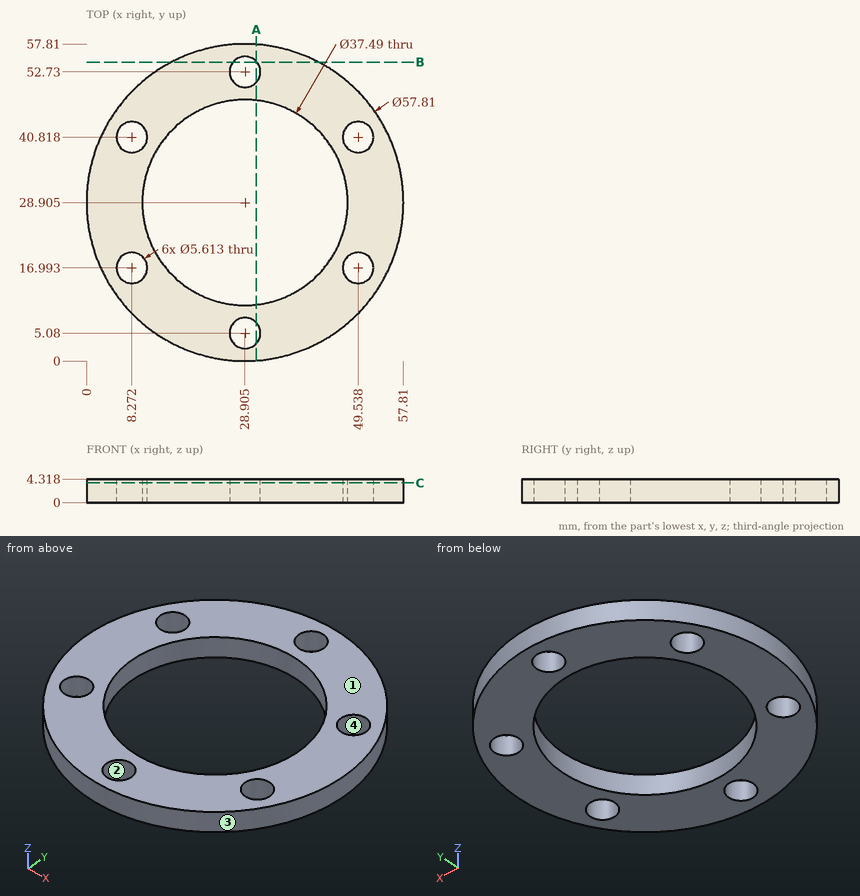
Check sheet for the drawn part. Datum: minimum x, y, z corner. Units: mm. Give positions to 0.01 mm unless a question says otherwise; leave off trailing zeros. Loops run counter-clockwise (first coordinate to the right, second up) from the corner with the lowest first, then second, coordinate; pieces in that order, holes last.
1) Depth check by flat-ended pin: pin 1 Ø1 at (y, z) = (49.5, 1.5) entering from -X; pin 2 Ø7.5 at (x, y) = (8.27, 40.82) entering from -Z; pin 3 Ø2 at (x, z) = (48, 2) entering from -Y (1 decimal); pin 4 Ø2 at (x, z) = (10, 1.5) entering from -Y. Enter the tip coordinate at first touch or a pass-through.
2) Draft check along X on the marked faces 1, 2, 3 and 4. Enter one of: pulls with the +X half, pulls with the -X half, needs draft (parallel to the pull), parting line crosses it, or undercut.
3) Sectioned sample at B-B, the plane y = 54.5. Enter the section's corners in (x, z).
4) Thickness scan on line 1 along Y through (x, z) = (28, 2.6) (1 decimal); line 2 along Y through (x, z) = (51, 2.85) (1 decimal); line 3 along Y through (x, z) = (30.5, 1.2) (1 decimal). Record the ranges inside material, lowest first.
5) Sectioned sample at A-A, the plane x = 31. Enter the section's corners in (y, z) (1 decimal).
6) Sectioned sample at C-C, the plane z = 3.6. Count the separate pieces of the cut face and the enclosed holes in it, then the cut area to 3 significant figures.
Answers:
1. pin 1: stops at x = 8.13
1. pin 2: stops at z = 0
1. pin 3: stops at y = 6.4
1. pin 4: stops at y = 6.21
2. face 1: needs draft
2. face 2: undercut
2. face 3: parting line crosses it
2. face 4: undercut
3. outline: (15.47, 0) - (26.73, 0) - (26.73, 4.32) - (15.47, 4.32) - close; (31.08, 0) - (42.34, 0) - (42.34, 4.32) - (31.08, 4.32) - close
4. line 1: y = 0 to 2.4, 7.7 to 10.2, 47.6 to 50.1, 55.4 to 57.8
4. line 2: y = 10.3 to 14.6, 19.4 to 38.4, 43.2 to 47.5
4. line 3: y = 0 to 2.8, 7.4 to 10.2, 47.6 to 50.4, 55 to 57.8
5. outline: (0.1, 0) - (3.2, 0) - (3.2, 4.3) - (0.1, 4.3) - close; (6.9, 0) - (10.3, 0) - (10.3, 4.3) - (6.9, 4.3) - close; (47.5, 0) - (50.9, 0) - (50.9, 4.3) - (47.5, 4.3) - close; (54.6, 0) - (57.7, 0) - (57.7, 4.3) - (54.6, 4.3) - close
6. separate pieces: 1
6. enclosed holes: 7
6. area: 1,370 mm2
